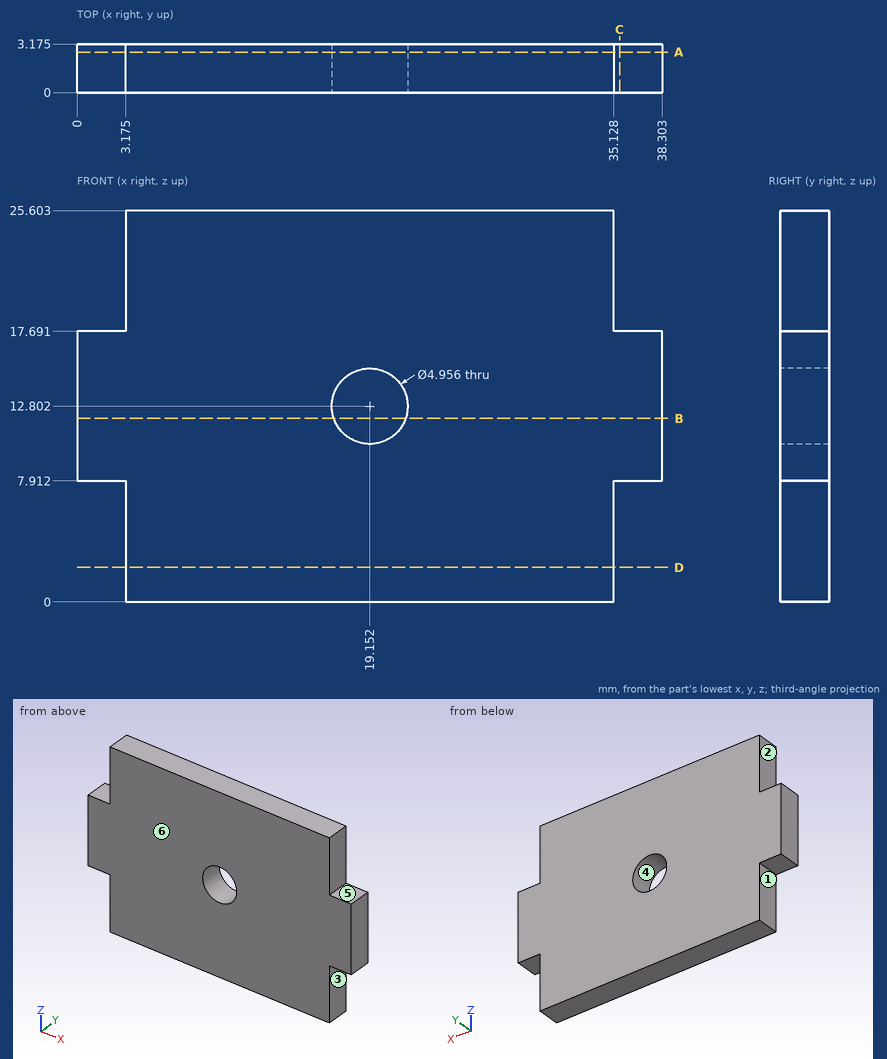
Could you check a few things on this drawing? It's one solid part, dimensions in mm from its lowest x, y, z. A direction names the side the tool comes from. Coordinates: 2 decimals unless noted, no trailing zeros. Write each loop counter-clockwise with the first axis right and the second up, starting at its lowest first coordinate (ties: lowest second). Pieces come first, ordered by that corner, then holes.
1) If we section it at A-A (y = 2.65): List the corners of the cut face in (x, z) for me (1 decimal).
Filled in:
outline: (0, 7.9) - (3.2, 7.9) - (3.2, 0) - (35.1, 0) - (35.1, 7.9) - (38.3, 7.9) - (38.3, 17.7) - (35.1, 17.7) - (35.1, 25.6) - (3.2, 25.6) - (3.2, 17.7) - (0, 17.7) - close; hole circle Ø5 at (19.2, 12.8)
2) If I drill on line 1 (X direction, y = 0.65, z = 12); line 2 (X direction, y = 1.2, z = 5.75) (1 decimal), over which ranges is the centre line in solid material (lowest first)?
Filled in:
line 1: x = 0 to 16.81, 21.5 to 38.3
line 2: x = 3.2 to 35.1
3) Which directions (+Z, -Z, +X, -X, +Y, -Y) give clear straight access to the entire face, cutting with the end or side of a thin tool? Please do the marked faces 1, 2 and 3.
Filled in:
face 1: -Z, -X, +Y, -Y
face 2: +Z, -X, +Y, -Y
face 3: -Z, +X, +Y, -Y
4) If we section it at B-B (z = 12): List the corners of the cut face in (x, y) for me (1 decimal), plus the area to 3 significant figures.
Filled in:
outline: (0, 0) - (16.8, 0) - (16.8, 3.2) - (0, 3.2) - close; (21.5, 0) - (38.3, 0) - (38.3, 3.2) - (21.5, 3.2) - close
area: 107 mm2
5) I'm going to push flat-ended pins straight in: pin 1 (1 mm diameter, centred on x = 1, y = 1, fed in from +Z); pin 2 (1.5 mm diameter, centred on y = 2.5, z = 8.5, fed in from -X); pin 3 (1.6 mm diameter, centred on y = 1, z = 22, fed in from -X) (3 decimals); pin 4 (1 mm diameter, centred on x = 36.5, y = 1.5, fed in from -Z). Where does each tip first touch, or does it pass through?
Filled in:
pin 1: stops at z = 17.69
pin 2: stops at x = 0
pin 3: stops at x = 3.175
pin 4: stops at z = 7.91
6) If we section it at D-D (z = 2.25): List the corners of the cut face in (x, y) for me (1 decimal).
Filled in:
outline: (3.2, 0) - (35.1, 0) - (35.1, 3.2) - (3.2, 3.2) - close
7) If we section it at C-C (x = 35.5): List the corners of the cut face in (y, z) for me (1 decimal).
Filled in:
outline: (0, 7.9) - (3.2, 7.9) - (3.2, 17.7) - (0, 17.7) - close
8) Thinking about a two-plate mould opening in Z: for the marked faces 4, 5 and 6, which applies, +Z half, -Z half, draft (parallel to the pull), parting line (faces both ways), or undercut?
Filled in:
face 4: undercut
face 5: +Z half
face 6: draft
